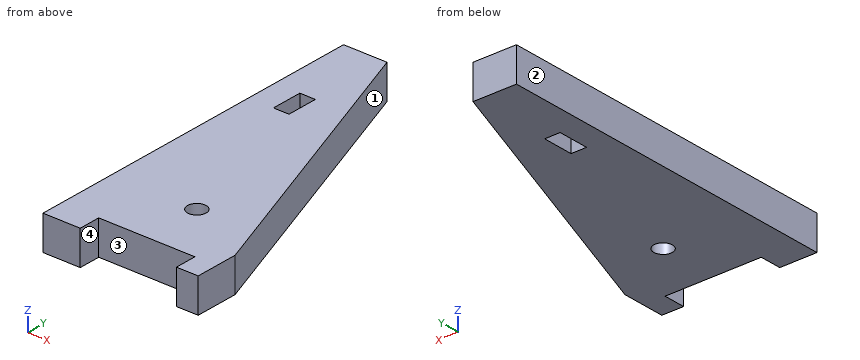
from build123d import *

# Parameters (mm, degrees)
SALIENTE_EXTRUIR1_DEPTH = 5.5
SALIENTE_EXTRUIR2_DEPTH = 5.5
CROQUIS3_W              = 15.5
CROQUIS3_H              = 3.5
CORTAR_EXTRUIR1_DEPTH   = 5.5
CROQUIS4_R              = 1.5
CORTAR_EXTRUIR2_DEPTH   = 5.5
CROQUIS5_W              = 2.5
CROQUIS5_H              = 5
CORTAR_EXTRUIR3_DEPTH   = 10


with BuildPart() as part:
    # Croquis1 → Saliente-Extruir1 (new body)
    with BuildSketch(Plane.XY):
        Polygon((0, 0), (0, -50), (25, -50), (25, -43), (7, -43), (7, 0), align=None)
    extrude(amount=SALIENTE_EXTRUIR1_DEPTH)

    # Croquis2 → Saliente-Extruir2 (add)
    with BuildSketch(Plane.XY.offset(5.5)):
        Polygon((25, -43), (0, -43), (0, 7), (7, 7), align=None)
    extrude(amount=-SALIENTE_EXTRUIR2_DEPTH)

    # Croquis3 → Cortar-Extruir1 (cut)
    with BuildSketch(Plane.XY.offset(5.5)):
        with Locations((13.75, -48.25)):
            Rectangle(CROQUIS3_W, CROQUIS3_H)
    extrude(amount=-CORTAR_EXTRUIR1_DEPTH, mode=Mode.SUBTRACT)

    # Croquis4 → Cortar-Extruir2 (cut)
    with BuildSketch(Plane.XY.offset(5.5)):
        with Locations((13.75, -37)):
            Circle(CROQUIS4_R)
    extrude(amount=-CORTAR_EXTRUIR2_DEPTH, mode=Mode.SUBTRACT)

    # Croquis5 → Cortar-Extruir3 (cut)
    with BuildSketch(Plane.XY.offset(5.5)):
        with Locations((5.25, -8.5)):
            Rectangle(CROQUIS5_W, CROQUIS5_H)
    extrude(amount=-CORTAR_EXTRUIR3_DEPTH, mode=Mode.SUBTRACT)


solid = part.part
Input: part model. Units: mm. Frame: model coordinates. Face numbers are marked on the shaded views. Round coordinates to 2 decimals unless told otherwise and drop trailing zeros. Order: outer loops, then holes, each group sorted by start corner. A loop starts at its lowest first (then second) coordinate and runs counter-clockwise, first axis right, second up. Notation, with made-up numbers: (-12, -10) - (29, -10) arc R28 ccw to (29, 16) - close; hole circle Ø9 at (17, -17.75). An arc over 180 degrees is marked (long way). Use a Markdown table: item, result.
1. Section B-B on x = 13.75. Return the cut outline in (y, z), then the cut area to 3 significant figures.
Evaluation:
| item | result |
|---|---|
| outline | (-46.5, 0) - (-38.5, 0) - (-38.5, 5.5) - (-46.5, 5.5) - close; (-35.5, 0) - (-11.75, 0) - (-11.75, 5.5) - (-35.5, 5.5) - close |
| area | 175 mm^2 |
2. Mould query, pull axis X, two halves, no side actions, for the marked faces 1, 2, 3 and 4. Classes: +X half, -X half, draft (parallel to the pull), parting line (faces both ways), or undercut.
Evaluation:
| item | result |
|---|---|
| face 1 | +X half |
| face 2 | -X half |
| face 3 | undercut |
| face 4 | undercut |
3. Section A-A on y = -37. Return the cut outline in (x, z).
Evaluation:
| item | result |
|---|---|
| outline | (0, 0) - (12.25, 0) - (12.25, 5.5) - (0, 5.5) - close; (15.25, 0) - (22.84, 0) - (22.84, 5.5) - (15.25, 5.5) - close |
4. First-contact query: pin 1 (1 mm diameter, centred on y = -2.5, z = 4, fed in from +X). Flat tip, straight axial feed; report the tip coordinate or a pass-through.
Evaluation:
| item | result |
|---|---|
| pin 1 | x = 10.6 |
5. Material intervals for probe 1 along X at (y, z) = (-10, 2.9); probe 2 along X at (y, z) = (-36, 5.2); probe 3 along X at (y, z) = (-22, 4.05), sorted ascending.
Evaluation:
| item | result |
|---|---|
| probe 1 | 0 to 4, 6.5 to 13.12 |
| probe 2 | 0 to 12.63, 14.87 to 22.48 |
| probe 3 | 0 to 17.44 |
6. Section D-D on y = -24.5. Return the cut outline in (x, z), then the cut area to 3 significant figures.
Evaluation:
| item | result |
|---|---|
| outline | (0, 0) - (18.34, 0) - (18.34, 5.5) - (0, 5.5) - close |
| area | 101 mm^2 |
7. Section C-C on z = 4.3. Return the cut outline in (x, y).
Evaluation:
| item | result |
|---|---|
| outline | (0, -50) - (6, -50) - (6, -46.5) - (21.5, -46.5) - (21.5, -50) - (25, -50) - (25, -43) - (7, 7) - (0, 7) - close; hole (4, -11) - (6.5, -11) - (6.5, -6) - (4, -6) - close; hole circle Ø3 at (13.75, -37) |
